from build123d import *

# Parameters (mm, degrees)
SKETCH001_W  = 9
SKETCH001_H  = 27
PAD001_DEPTH = 3
SKETCH_W     = 45.8
SKETCH_H     = 47
PAD_DEPTH    = 3
SKETCH002_W  = 9
SKETCH002_H  = 27
PAD002_DEPTH = 3
FILLET_R     = 1
FILLET001_R  = 3


with BuildPart() as pad001:
    # Sketch001 → Pad001 (new body)
    with BuildSketch(Plane.YZ.offset(3)):
        with Locations((42.5, 13.5)):
            Rectangle(SKETCH001_W, SKETCH001_H)
        with BuildLine():
            ThreePointArc((44.1, 22), (42.5, 23.6), (40.9, 22))
            Line((40.9, 22), (40.9, 6))
            ThreePointArc((40.9, 6), (42.5, 4.4), (44.1, 6))
            Line((44.1, 22), (44.1, 6))
        make_face(mode=Mode.SUBTRACT)
    extrude(amount=-PAD001_DEPTH)


with BuildPart() as fusion:
    # Sketch → Pad (new body)
    with BuildSketch(Plane.XY):
        with Locations((22.9, 23.5)):
            Rectangle(SKETCH_W, SKETCH_H)
        Polygon((7.3, 44), (10.5, 44), (10.5, 30.5), (14.4, 30.5), (14.4, 44), (31.4, 44), (31.4, 30.5), (35.3, 30.5), (35.3, 44), (38.5, 44), (38.5, 3), (35.3, 3), (35.3, 16.5), (31.4, 16.5), (31.4, 3), (14.4, 3), (14.4, 16.5), (10.5, 16.5), (10.5, 3), (7.3, 3), align=None, mode=Mode.SUBTRACT)
    extrude(amount=PAD_DEPTH)

    # Fusion: union Pad001
    add(pad001.part)


with BuildPart() as fillet001:
    # Sketch002 → Pad002 (new body)
    with BuildSketch(Plane.YZ.offset(45.8)):
        with Locations((42.5, 13.5)):
            Rectangle(SKETCH002_W, SKETCH002_H)
        with BuildLine():
            ThreePointArc((44.1, 22), (42.5, 23.6), (40.9, 22))
            Line((40.9, 22), (40.9, 6))
            ThreePointArc((40.9, 6), (42.5, 4.4), (44.1, 6))
            Line((44.1, 22), (44.1, 6))
        make_face(mode=Mode.SUBTRACT)
    extrude(amount=-PAD002_DEPTH)

    # Fusion001: union Fusion
    add(fusion.part)

    # Fillet
    fillet_edges = [fillet001.edges().sort_by_distance(p)[0] for p in [
        (1.5, 38, 3),
        (3, 42.5, 3),
        (42.8, 42.5, 3),
        (44.3, 38, 3),
    ]]
    fillet(fillet_edges, radius=FILLET_R)

    # Fillet001
    fillet001_edges = [fillet001.edges().sort_by_distance(p)[0] for p in [
        (1.5, 38, 27),
        (44.3, 38, 27),
        (1.5, 47, 27),
        (44.3, 47, 27),
    ]]
    fillet(fillet001_edges, radius=FILLET001_R)


solid = fillet001.part
Read the model definition and answer for the solid it produces. Units are mm, in the model's axes. A direction names the side the tool comes from. Give positions to 0.01 mm unless a question says otherwise; leave off trailing zeros. Write each loop counter-clockwise with the first axis right and the second up, starting at its lowest first coordinate (ties: lowest second). Pieces come first, ordered by that corner, then holes. Notation, with made-up numbers: (49, 60.25) - (67, 60.25) arc R25 ccw to (67, 75.25) - close; hole circle Ø3 at (-17, 39.5). An arc over 180 degrees is marked (long way). Use CSV: the item, a comma, the result in double quotes. Start each with the question number.
Item 1: Consider line 1 (Y direction, x = 13, z = 2.5); line 2 (X direction, y = 41, z = 4.75); line 3 (Y direction, x = 43, z = 6.5). Determine where each line is inside the solid, lowest interval first.
Item 2: The mould has two halves that part along X. Classify faces 6 (the flat face through (33, 30.5, 1)), 7 (the flat face through (23, 47, 2)), 8 (the flat face through (0, 39, 9)): pulls with the +X half, pulls with the -X half, needs draft (parallel to the pull), parting line crosses it, or undercut.
Item 3: For faces 1 (the flat face through (3, 40, 16)), 2 (the flat face through (37, 44, 1)), 3 (the flat face through (44, 40.9, 14)), 4 (the flat face through (2, 38, 14)), 5 (the cylindrical face through (44.28, 46.14, 26.1)), determine the directions among +Z, -Z, +X, -X, +Y, -Y from which every point of the face is accessible in a straight line to the end or side of a thin tool.
Item 4: The part is cut by section B-B, the plane y = 35. Give the vertices of the cut face in (x, z), and give its area (3 significant figures).
Item 5: The part is cut by section D-D, the plane z = 24.75. Give the vertices of the cut face in (x, y), and give its area (3 significant figures).
Item 6: The part is cut by section C-C, the plane y = 42.5. Count the separate pieces of the cut face and the enclosed holes in it, and give its area (3 significant figures).
Item 7: A flat-ended cylindrical pin translates along its axis: P1, Ø12, axis at x = 7, z = 22, coming from the -Y side. Find the tip coordinate at first contact, or state that the pin passes through.
Item 8: The part is cut by section A-A, the plane x = 24.5. Give the vertices of the cut face in (y, z), and give its area (3 significant figures).
Taken from the geometry:
1,line 1,"0 to 16.5, 30.5 to 47"
1,line 2,"0 to 3, 42.8 to 45.8"
1,line 3,"38 to 40.9, 44.1 to 47"
2,face 6,"undercut"
2,face 7,"needs draft"
2,face 8,"pulls with the -X half"
3,face 1,"+Z, +Y, -Y"
3,face 2,"+Z, -Z"
3,face 3,"+X, -X"
3,face 4,"+Z, +X, -X, -Y"
3,face 5,"+Z, +X, -X, +Y"
4,outline,"(0, 0) - (7.3, 0) - (7.3, 3) - (0, 3) - close; (10.5, 0) - (14.4, 0) - (14.4, 3) - (10.5, 3) - close; (31.4, 0) - (35.3, 0) - (35.3, 3) - (31.4, 3) - close; (38.5, 0) - (45.8, 0) - (45.8, 3) - (38.5, 3) - close"
4,area,"67.2 mm2"
5,outline,"(0, 38.1) - (3, 38.1) - (3, 46.9) - (0, 46.9) - close; (42.8, 38.1) - (45.8, 38.1) - (45.8, 46.9) - (42.8, 46.9) - close"
5,area,"52.9 mm2"
6,separate pieces,"6"
6,enclosed holes,"0"
6,area,"96.4 mm2"
7,P1,"y = 38"
8,outline,"(0, 0) - (3, 0) - (3, 3) - (0, 3) - close; (44, 0) - (47, 0) - (47, 3) - (44, 3) - close"
8,area,"18.0 mm2"
